from build123d import *

# Parameters (mm, degrees)
SKETCH_1_W      = 400
SKETCH_1_H      = 14
SKETCH_1_R      = 2.6
SKETCH_1_R_2    = 1.1
EXTRUDE_1_DEPTH = 2
CHAMFER_1_SIZE  = 1.9


with BuildPart() as part:
    # Эскиз1 → Вытянуть1 (new body)
    with BuildSketch(Plane.XY):
        Rectangle(SKETCH_1_W, SKETCH_1_H)
        with Locations(Location((-180, 0, 0), (0, 0, 180))):
            Circle(SKETCH_1_R, mode=Mode.SUBTRACT)
        with Locations(Location((-100, 0, 0), (0, 0, 180))):
            Circle(SKETCH_1_R, mode=Mode.SUBTRACT)
        with Locations(Location((-20, 0, 0), (0, 0, 180))):
            Circle(SKETCH_1_R, mode=Mode.SUBTRACT)
        with Locations(Location((20, 0, 0), (0, 0, 180))):
            Circle(SKETCH_1_R, mode=Mode.SUBTRACT)
        with Locations(Location((100, 0, 0), (0, 0, 180))):
            Circle(SKETCH_1_R, mode=Mode.SUBTRACT)
        with Locations(Location((180, 0, 0), (0, 0, 180))):
            Circle(SKETCH_1_R, mode=Mode.SUBTRACT)
        with Locations((-196, -1)):
            Circle(SKETCH_1_R_2, mode=Mode.SUBTRACT)
        with Locations((-4, -1)):
            Circle(SKETCH_1_R_2, mode=Mode.SUBTRACT)
        with Locations(Location((4, -1, 0), (0, 0, 180))):
            Circle(SKETCH_1_R_2, mode=Mode.SUBTRACT)
        with Locations(Location((196, -1, 0), (0, 0, 180))):
            Circle(SKETCH_1_R_2, mode=Mode.SUBTRACT)
    extrude(amount=EXTRUDE_1_DEPTH)

    # Фаска1
    chamfer_1_edges = [part.edges().sort_by_distance(p)[0] for p in [
        (-177.4, 0, 2),
        (-97.4, 0, 2),
        (-17.4, 0, 2),
        (22.6, 0, 2),
        (102.6, 0, 2),
        (182.6, 0, 2),
    ]]
    chamfer(chamfer_1_edges, length=CHAMFER_1_SIZE)


solid = part.part
Geometry: final body of the model. Coordinates: model frame, mm. Give positions to 0.01 mm unless a question says otherwise; leave off trailing zeros. Put each result on its own line as item: value.
1) Mould query, pull axis X, two halves, no side actions, for faces 1 (the conical face through (182.72, -0.12, 0.22)), 2 (the flat face through (-3, 0, 2)). Classes: released by +X, released by -X, zero draft, split by the parting line, or undercut.
Computed values:
face 1: undercut
face 2: zero draft
2) First-contact query: P1, Ø3, axis at x = 180, y = 0, coming from the +Z side; P2, Ø3.5, axis at x = 4, y = -1, coming from the +Z side; P3, Ø6, axis at x = 20, y = 0, coming from the +Z side. Flat tips, straight axial feed; report the tip coordinate or a pass-through.
Computed values:
P1: passes through
P2: stops at z = 2
P3: stops at z = 0.5
3) Cut plane A-A, the plane z = 1.3. Give the number of separate pieces and of enclosed holes in the cut face, plus the area to 3 significant figures.
Computed values:
separate pieces: 1
enclosed holes: 10
area: 5,310 mm^2
4) Material intervals for L1, parallel to Y at x = 196, z = 0.95; L2, parallel to Y at x = -100, z = 0.05, sorted ascending. Write a range as from..to.
Computed values:
L1: y = -7..-2.1, 0.1..7
L2: y = -7..-2.6, 2.6..7
